Input: part model. Units: mm. Frame: model coordinates. Face numbers are marked on the shaded views. A direction names the side the tool comes from. Coordinates: 2 decimals unless noted, no trailing zeros. Loops run counter-clockwise (first coordinate to the right, second up) from the corner with the lowest first, then second, coordinate; pieces in that order, holes last. Notation, with made-up numbers: (69, 39) - (110, 39) arc R23 ccw to (110, 68) - close; hole circle Ø7 at (-28.75, 69.25). An arc over 180 degrees is marked (long way). Use a Markdown table: item, result. Add a question column.
1. Section query D-D on y = 8. Return the cut outline in (x, z).
2. Section query B-B on z = 2. Return the cut outline in (x, y).
3. Access query for the marked faces 1, 2 and 3. Directions: +Z, -Z, +X, -X, +Y, -Y. A direction counts if a zero-diameter tool reaches every point of the face in a straight line with its end or side. Return the directions, or none.
4. Draft query along Y for the marked faces 4, 5, 6 and 7. Return one class per face: released by +Y, released by -Y, zero draft, split by the parting line, or undercut.
5. Section query C-C on x = 10. Return the cut outline in (y, z).
6. Section query A-A on x = 0. Return the cut outline in (y, z).
7. Ray query, L1, parallel to X at y = 0, z = 1; L2, parallel to X at y = 5.5, z = 2.25; L3, parallel to Y at x = -2.5, z = 0.75. Return the intervals inside material, ascending. Write a range as [from, to].
8. Contact query for flat-ended pins moving along their axis: P1, Ø2, axis at x = -10.5, z = 1, coming from the +Y side; P2, Ø3, axis at x = -13.86, y = 8, coming from the +Z side; P3, Ø2, axis at x = -5.5, z = -3, coming from the +Y side; P4, Ø3, axis at x = 8.5, z = -1.5, coming from the -Y side. Output: stop coordinate, or through.
```python
from build123d import *

# Parameters (mm, degrees)
CORTAR_EXTRUIR1_DEPTH = 7
CORTAR_EXTRUIR2_REACH = 30.443
CROQUIS5_R            = 1.6


with BuildPart() as part:
    # Croquis1 → Revolución1 (revolve)
    with BuildSketch(Plane(origin=(0, 0, 0), x_dir=(1, 0, 0), z_dir=(0, 1, 0))):
        Polygon((-12, 4.5), (-19.3, 4.5), (-19.3, 3.5), (-17.5, 3.5), (-17.5, -3.5), (-12, -3.5), align=None)
    revolve(axis=Axis((0, 0, -14.909787419), (0, 0, 1)))

    # Croquis2 → Cortar-Extruir1 (cut)
    with BuildSketch(Plane.XY.offset(3.5)):
        with BuildLine():
            Line((1.6, 16), (1.6, 17.426703647))
            ThreePointArc((1.6, 17.426703647), (0, 17.5), (-1.6, 17.426703647))
            Line((-1.6, 17.426703647), (-1.6, 16))
            ThreePointArc((-1.6, 16), (0, 14.4), (1.6, 16))
        make_face()
        with BuildLine():
            Line((14.656406461, 6.614359354), (15.891968063, 7.327711177))
            ThreePointArc((15.891968063, 7.327711177), (15.155444566, 8.75), (14.291968063, 10.09899247))
            Line((14.291968063, 10.09899247), (13.056406461, 9.385640646))
            ThreePointArc((13.056406461, 9.385640646), (12.470765814, 7.2), (14.656406461, 6.614359354))
        make_face()
        with BuildLine():
            Line((13.056406461, -9.385640646), (14.291968063, -10.09899247))
            ThreePointArc((14.291968063, -10.09899247), (15.155444566, -8.75), (15.891968063, -7.327711177))
            Line((15.891968063, -7.327711177), (14.656406461, -6.614359354))
            ThreePointArc((14.656406461, -6.614359354), (12.470765814, -7.2), (13.056406461, -9.385640646))
        make_face()
        with BuildLine():
            Line((-1.6, -16), (-1.6, -17.426703647))
            ThreePointArc((-1.6, -17.426703647), (0, -17.5), (1.6, -17.426703647))
            Line((1.6, -17.426703647), (1.6, -16))
            ThreePointArc((1.6, -16), (0, -14.4), (-1.6, -16))
        make_face()
        with BuildLine():
            Line((-14.656406461, -6.614359354), (-15.891968063, -7.327711177))
            ThreePointArc((-15.891968063, -7.327711177), (-15.155444566, -8.75), (-14.291968063, -10.09899247))
            Line((-14.291968063, -10.09899247), (-13.056406461, -9.385640646))
            ThreePointArc((-13.056406461, -9.385640646), (-12.470765814, -7.2), (-14.656406461, -6.614359354))
        make_face()
        with BuildLine():
            Line((-13.056406461, 9.385640646), (-14.291968063, 10.09899247))
            ThreePointArc((-14.291968063, 10.09899247), (-15.155444566, 8.75), (-15.891968063, 7.327711177))
            Line((-15.891968063, 7.327711177), (-14.656406461, 6.614359354))
            ThreePointArc((-14.656406461, 6.614359354), (-12.470765814, 7.2), (-13.056406461, 9.385640646))
        make_face()
    extrude(amount=-CORTAR_EXTRUIR1_DEPTH, mode=Mode.SUBTRACT)

    # Croquis5 → Cortar-Extruir2 (cut, up to next)
    with BuildSketch(Plane(origin=(0, 0, -4.5), x_dir=(-1, 0, 0), z_dir=(0, 0, -1)), mode=Mode.PRIVATE) as cortar_extruir2_sk1:
        with Locations((0, 16)):
            Circle(CROQUIS5_R)
    cortar_extruir2_tool1 = extrude(cortar_extruir2_sk1.sketch, amount=-CORTAR_EXTRUIR2_REACH, mode=Mode.PRIVATE) & part.part
    # Croquis5 → Cortar-Extruir2 (cut, up to next)
    with BuildSketch(Plane(origin=(0, 0, -4.5), x_dir=(-1, 0, 0), z_dir=(0, 0, -1)), mode=Mode.PRIVATE) as cortar_extruir2_sk2:
        with Locations(Location((13.856406461, 8, 0), (0, 0, 120))):
            Circle(CROQUIS5_R)
    cortar_extruir2_tool2 = extrude(cortar_extruir2_sk2.sketch, amount=-CORTAR_EXTRUIR2_REACH, mode=Mode.PRIVATE) & part.part
    # Croquis5 → Cortar-Extruir2 (cut, up to next)
    with BuildSketch(Plane(origin=(0, 0, -4.5), x_dir=(-1, 0, 0), z_dir=(0, 0, -1)), mode=Mode.PRIVATE) as cortar_extruir2_sk3:
        with Locations(Location((13.856406461, -8, 0), (0, 0, 240))):
            Circle(CROQUIS5_R)
    cortar_extruir2_tool3 = extrude(cortar_extruir2_sk3.sketch, amount=-CORTAR_EXTRUIR2_REACH, mode=Mode.PRIVATE) & part.part
    # Croquis5 → Cortar-Extruir2 (cut, up to next)
    with BuildSketch(Plane(origin=(0, 0, -4.5), x_dir=(-1, 0, 0), z_dir=(0, 0, -1)), mode=Mode.PRIVATE) as cortar_extruir2_sk4:
        with Locations((0, -16)):
            Circle(CROQUIS5_R)
    cortar_extruir2_tool4 = extrude(cortar_extruir2_sk4.sketch, amount=-CORTAR_EXTRUIR2_REACH, mode=Mode.PRIVATE) & part.part
    # Croquis5 → Cortar-Extruir2 (cut, up to next)
    with BuildSketch(Plane(origin=(0, 0, -4.5), x_dir=(-1, 0, 0), z_dir=(0, 0, -1)), mode=Mode.PRIVATE) as cortar_extruir2_sk5:
        with Locations(Location((-13.856406461, -8, 0), (0, 0, 120))):
            Circle(CROQUIS5_R)
    cortar_extruir2_tool5 = extrude(cortar_extruir2_sk5.sketch, amount=-CORTAR_EXTRUIR2_REACH, mode=Mode.PRIVATE) & part.part
    # Croquis5 → Cortar-Extruir2 (cut, up to next)
    with BuildSketch(Plane(origin=(0, 0, -4.5), x_dir=(-1, 0, 0), z_dir=(0, 0, -1)), mode=Mode.PRIVATE) as cortar_extruir2_sk6:
        with Locations(Location((-13.856406461, 8, 0), (0, 0, 240))):
            Circle(CROQUIS5_R)
    cortar_extruir2_tool6 = extrude(cortar_extruir2_sk6.sketch, amount=-CORTAR_EXTRUIR2_REACH, mode=Mode.PRIVATE) & part.part
    add(cortar_extruir2_tool1.solids().sort_by_distance((0, 16, -4.5))[0], mode=Mode.SUBTRACT)
    add(cortar_extruir2_tool2.solids().sort_by_distance((-13.856406, 8, -4.5))[0], mode=Mode.SUBTRACT)
    add(cortar_extruir2_tool3.solids().sort_by_distance((-13.856406, -8, -4.5))[0], mode=Mode.SUBTRACT)
    add(cortar_extruir2_tool4.solids().sort_by_distance((0, -16, -4.5))[0], mode=Mode.SUBTRACT)
    add(cortar_extruir2_tool5.solids().sort_by_distance((13.856406, -8, -4.5))[0], mode=Mode.SUBTRACT)
    add(cortar_extruir2_tool6.solids().sort_by_distance((13.856406, 8, -4.5))[0], mode=Mode.SUBTRACT)


solid = part.part
```
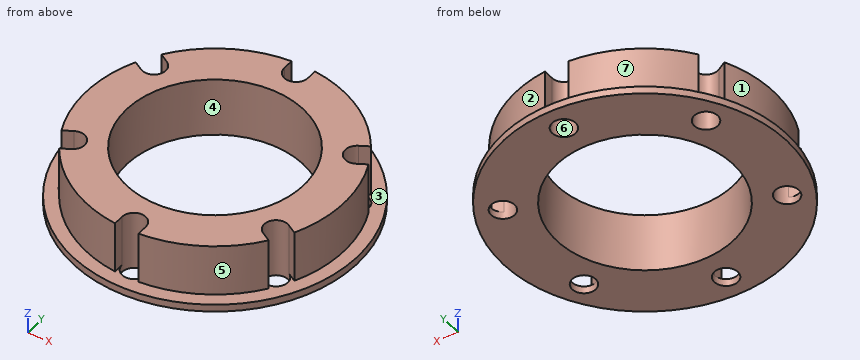
Resolved:
| question | item | result |
|---|---|---|
| 1 | outline | (-17.56, -4.5) - (-15.46, -4.5) - (-15.46, -3.5) - (-17.56, -3.5) - close; (-12.26, -4.5) - (-8.94, -4.5) - (-8.94, 3.5) - (-12.26, 3.5) - close; (8.94, -4.5) - (12.26, -4.5) - (12.26, 3.5) - (8.94, 3.5) - close; (15.46, -4.5) - (17.56, -4.5) - (17.56, -3.5) - (15.46, -3.5) - close |
| 2 | outline | (-15.89, -7.33) - (-14.66, -6.61) arc R1.6 cw to (-13.06, -9.39) - (-14.29, -10.1) arc R17.5 ccw to (-1.6, -17.43) - (-1.6, -16) arc R1.6 cw to (1.6, -16) - (1.6, -17.43) arc R17.5 ccw to (14.29, -10.1) - (13.06, -9.39) arc R1.6 cw to (14.66, -6.61) - (15.89, -7.33) arc R17.5 ccw to (15.89, 7.33) - (14.66, 6.61) arc R1.6 cw to (13.06, 9.39) - (14.29, 10.1) arc R17.5 ccw to (1.6, 17.43) - (1.6, 16) arc R1.6 cw to (-1.6, 16) - (-1.6, 17.43) arc R17.5 ccw to (-14.29, 10.1) - (-13.06, 9.39) arc R1.6 cw to (-14.66, 6.61) - (-15.89, 7.33) arc R17.5 ccw to start; hole circle Ø24 at (0, 0) |
| 3 | face 1 | +Z, -X |
| 3 | face 2 | +Z, +X, +Y |
| 3 | face 3 | +Z |
| 4 | face 4 | undercut |
| 4 | face 5 | released by -Y |
| 4 | face 6 | undercut |
| 4 | face 7 | released by +Y |
| 5 | outline | (-16.51, -4.5) - (-6.63, -4.5) - (-6.63, 3.5) - (-14.36, 3.5) - (-14.36, -3.5) - (-16.51, -3.5) - close; (6.63, -4.5) - (16.51, -4.5) - (16.51, -3.5) - (14.36, -3.5) - (14.36, 3.5) - (6.63, 3.5) - close |
| 6 | outline | (-19.3, -4.5) - (-17.6, -4.5) - (-17.6, -3.5) - (-19.3, -3.5) - close; (-14.4, -4.5) - (-12, -4.5) - (-12, 3.5) - (-14.4, 3.5) - close; (12, -4.5) - (14.4, -4.5) - (14.4, 3.5) - (12, 3.5) - close; (17.6, -4.5) - (19.3, -4.5) - (19.3, -3.5) - (17.6, -3.5) - close |
| 7 | L1 | [-17.5, -12], [12, 17.5] |
| 7 | L2 | [-16.61, -10.67], [10.67, 16.61] |
| 7 | L3 | [-17.32, -11.74], [11.74, 17.32] |
| 8 | P1 | y = 14.7 |
| 8 | P2 | through |
| 8 | P3 | y = 18.74 |
| 8 | P4 | y = -16.04 |
